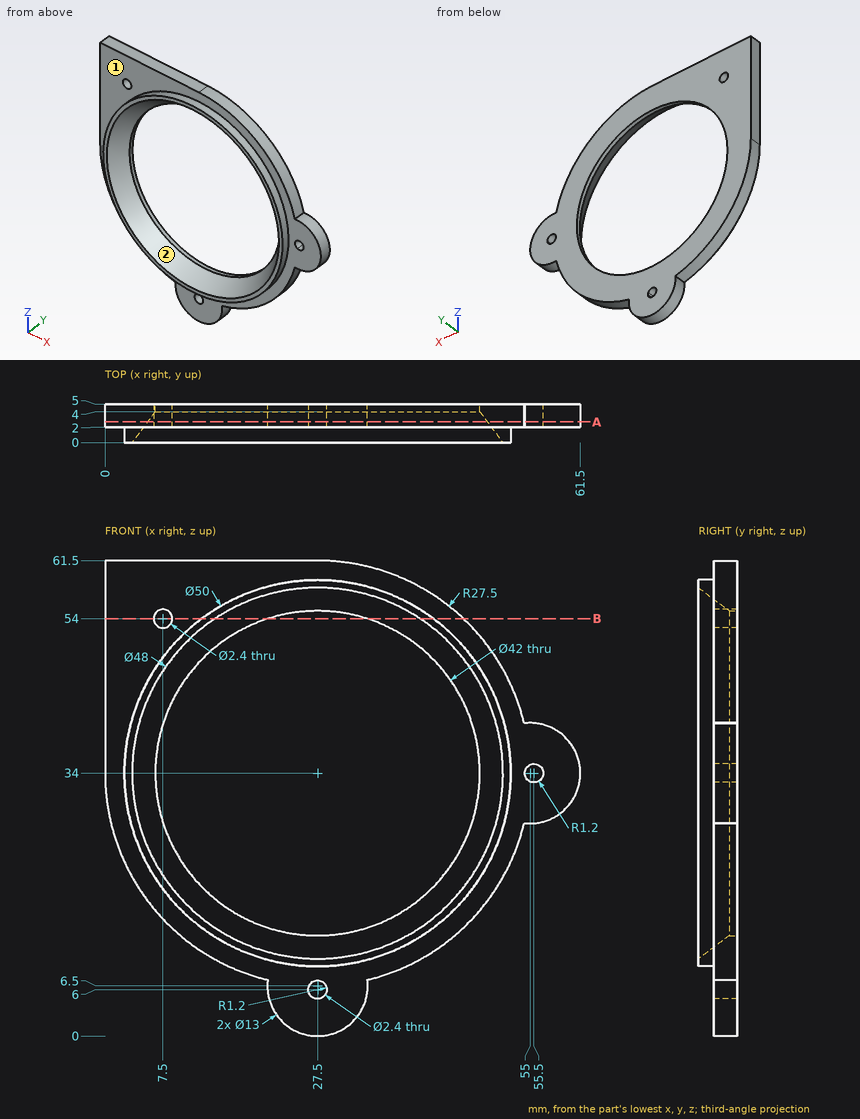
Can you work these out from the drawing? Everything is in mm from the part's minimum corner. Give positions to 0.01 mm unless a question says otherwise; leave off trailing zeros. Write each loop counter-clockwise with the first axis right and the second up, starting at its lowest first coordinate (ties: lowest second). Pieces come first, ordered by that corner, then holes. Notation, with made-up numbers: M 8.25,24.5 L 32.25,24.5 A11 ccw 32.25,30.5 Z; hole C 7,46 d10. An arc over 180 degrees is marked long. Answer in a Markdown table with one row per item. Add a question column.
Item 1: For pin 1 Ø12 at (x, z) = (43, 47) entering from +Y; pin 2 Ø1.5 at (y, z) = (2, 44.5) entering from +X; pin 3 Ø2 at (x, y) = (18, 2.5) entering from -Z, each with a flat end and sliding along its axis, tell me the tip position at first contact or that it passes through.
Item 2: Imagine slicing it at A-A, the plane y = 2.7. Write out the boundary of the cut face in (x, z) (3 decimals).
Item 3: We'd pull the mould along X, two halves only. Please class the marked faces 1 and 2: released by +X, released by -X, zero draft, split by the parting line, or undercut.
Item 4: Imagine slicing it at B-B, the plane z = 54. State how many separate pieces and enclosed holes the cut face has, plus the area to 3 significant figures.
Item 5: Please list where these lines run through material, in increasing order: L1, parallel to X at y = 4.65, z = 34; L2, parallel to Z at x = 27.5, y = 3.7 (3 decimals); L3, parallel to Z at x = 27.5, y = 3.3 (3 decimals).
Evaluation:
| question | item | result |
|---|---|---|
| 1 | pin 1 | stops at y = 5 |
| 1 | pin 2 | stops at x = 53.21 |
| 1 | pin 3 | stops at z = 7.85 |
| 2 | outline | M 0,34 A27.5 ccw 21.046,7.268 A6.5 ccw long 33.954,7.268 A27.5 ccw 54.232,27.546 A6.5 ccw long 54.232,40.454 A27.5 ccw 27.5,61.5 L 0,61.5 Z; hole C 27.5,34 d43.95; hole C 7.5,54 d2.4; hole M 28.581,6.521 A1.2 ccw long 28.7,6 A1.2 ccw Z; hole M 54.979,32.919 A1.2 ccw 56.7,34 A1.2 ccw 54.979,35.081 A1.2 ccw Z |
| 3 | face 1 | zero draft |
| 3 | face 2 | undercut |
| 4 | separate pieces | 3 |
| 4 | enclosed holes | 0 |
| 4 | area | 97.8 mm² |
| 5 | L1 | x = 0 to 6.5, 48.5 to 54.3, 56.7 to 61.5 |
| 5 | L2 | z = 0 to 4.8, 7.2 to 12.775, 55.225 to 61.5 |
| 5 | L3 | z = 0 to 4.8, 7.2 to 12.475, 55.525 to 61.5 |
